The model under review builds one solid part; all positions refer to its coordinate system, in mm. Face numbers are marked on the shaded views. Coordinates: 2 decimals unless noted, no trailing zeros. Order: outer loops, then holes, each group sorted by start corner. A loop starts at its lowest first (then second) coordinate and runs counter-clockwise, first axis right, second up.
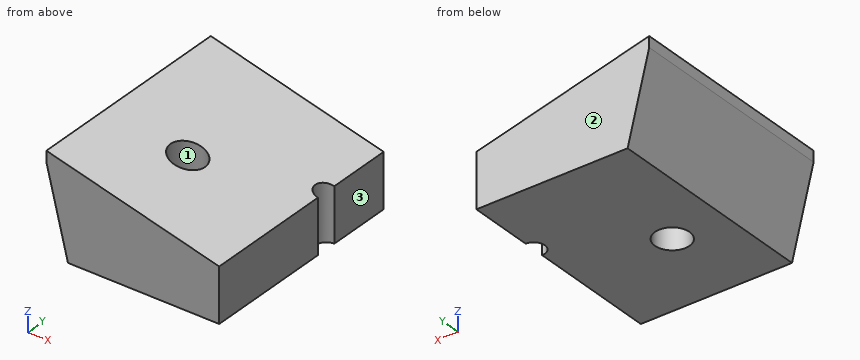
```python
from build123d import *

# Parameters (mm, degrees)
F1_DEPTH = 100
F2_R     = 8
F3_DEPTH = 45.001
F4_R     = 5
F5_DEPTH = 45.001


with BuildPart() as f1:
    # F0 (on Front) → F1 (new body)
    with BuildSketch(Plane.XZ):
        Polygon((-10, 40), (0, 0), (70, 0), (70, 25), (-10, 45), align=None)
    extrude(amount=-F1_DEPTH)

    # F2 (on face) → F3 (cut, through all)
    with BuildSketch(Plane(origin=(0, 0, 0), x_dir=(1, 0, 0), z_dir=(0, 0, -1))):
        with Locations((25, -40)):
            Circle(F2_R)
    extrude(amount=-F3_DEPTH, mode=Mode.SUBTRACT)

    # F4 (on face) → F5 (cut, through all)
    with BuildSketch(Plane(origin=(0, 0, 0), x_dir=(1, 0, 0), z_dir=(0, 0, -1))):
        with Locations((70, -65)):
            Circle(F4_R)
    extrude(amount=-F5_DEPTH, mode=Mode.SUBTRACT)


solid = f1.part
```
(1) For pin 1 Ø3 at (y, z) = (22, 20) entering from -X (3 decimals); pin 2 Ø13 at (x, y) = (25, 40) entering from +Z, all flat-tipped, find the tip position at first contact; note any pin that passes through.
A:
pin 1: stops at x = -5.375
pin 2: passes through
(2) We need section D-D, the plane y = 86. Write out the cut boundary in (x, z).
A:
outline: (-10, 40) - (0, 0) - (70, 0) - (70, 25) - (-10, 45) - close
(3) We need section A-A, the plane x = 25. Write out the cut boundary in (y, z), and give its area (4 significant figures).
A:
outline: (0, 0) - (32, 0) - (32, 36.25) - (0, 36.25) - close; (48, 0) - (100, 0) - (100, 36.25) - (48, 36.25) - close
area: 3,045 mm2
(4) We need section B-B, the plane z = 13. Write out the cut boundary in (x, y), and give its area (3 significant figures).
A:
outline: (-3.25, 0) - (70, 0) - (70, 60) arc R5 cw to (70, 70) - (70, 100) - (-3.25, 100) - close; hole circle Ø16 at (25, 40)
area: 7,080 mm2
(5) Wall thickness on probe 1 along Y at (x, z) = (25, 18); probe 2 along X at (y, z) = (40, 21); probe 3 along X at (y, z) = (40, 20): over which ranges is each line inside the solid? List them lowest first.
A:
probe 1: y = 0 to 32, 48 to 100
probe 2: x = -5.25 to 17, 33 to 70
probe 3: x = -5 to 17, 33 to 70
(6) Draft analysis for pull direction Y (two halves, no side actions). For the marked faces 1, 2 and 3, state which applies: released by +Y, released by -Y, zero draft, split by the parting line, or undercut.
A:
face 1: undercut
face 2: released by +Y
face 3: zero draft
(7) We need section C-C, the plane y = 40. Write out the cut boundary in (x, z), and give its area (3 significant figures).
A:
outline: (-10, 40) - (0, 0) - (17, 0) - (17, 38.25) - (-10, 45) - close; (33, 0) - (70, 0) - (70, 25) - (33, 34.25) - close
area: 2,020 mm2
